The drawing under review shows one solid part. Ordinate dimensions are in mm from its lowest x, y, z. Give positions to 0.01 mm unless a question says otherwise; leave off trailing zeros. Order: outer loops, then holes, each group sorted by start corner. A loop starts at its lowest first (then second) coordinate and runs counter-clockwise, first axis right, second up. Notation, with made-up numbers: (-30, -10.5) -> (-5, -10.5) arc R20 cw to (-5, 13.5) -> close; hole circle Ø11 at (86, -33). An arc over 180 degrees is marked (long way). One line per item, written item: value. Start each with the question number.
1) Consider section A-A (y = 1.25). State the section outline as (x, z) points, plus the area to 3 significant figures.
2) Consider section B-B (x = 60). State the section outline as (y, z) points.
3) Wall thickness on line 1 along Z through (x, y) = (40.5, 0.95); line 2 along X through (y, z) = (2.4, 8) (1 decimal); line 3 along X through (y, z) = (1.85, 182): over which ranges is each line inside the solid? List them lowest first. Write a range as from..to.
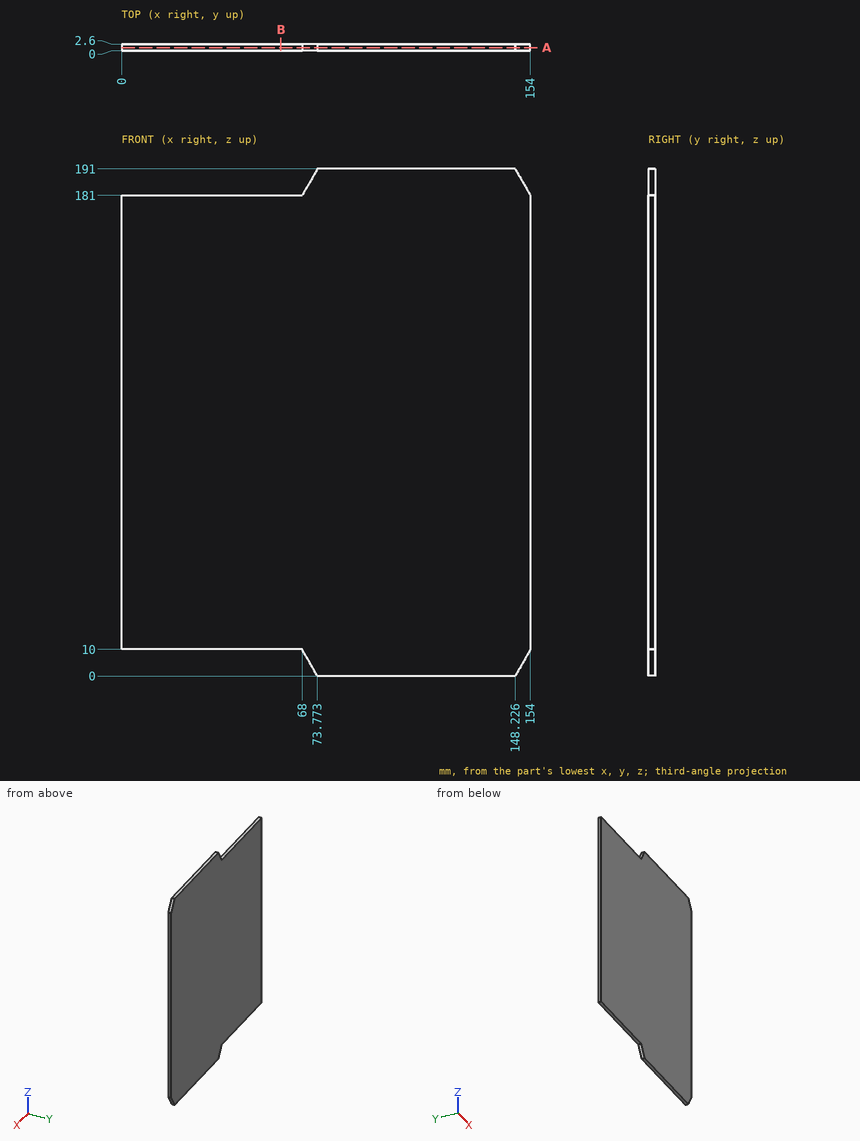
Checked values:
1. outline: (0, 10) -> (68, 10) -> (73.77, 0) -> (148.23, 0) -> (154, 10) -> (154, 181) -> (148.23, 191) -> (73.77, 191) -> (68, 181) -> (0, 181) -> close
1. area: 27,900 mm^2
2. outline: (0, 10) -> (2.6, 10) -> (2.6, 181) -> (0, 181) -> close
3. line 1: z = 10..181
3. line 2: x = 69.2..152.8
3. line 3: x = 68.58..153.42
